Source: CAD feature listing. Evaluate the final solid. Frame: model axes, mm. A direction names the side the tool comes from. Give positions to 0.01 mm unless a question says otherwise; leave off trailing zeros. Order: outer loops, then holes, each group sorted by start corner. A loop starts at its lowest first (then second) coordinate and runs counter-clockwise, first axis right, second up. Notation, with made-up numbers: M 22.25,57 L 40.25,57 A16 cw 40.25,82 Z; hole C 39.25,62.25 d11. An arc over 180 degrees is marked long. Answer as a JSON object with one key per item and string values. Group by question number.
1. Section query C-C (x = 19). Output: boundary loops of the cut face in (y, z).
2. Pin query (flat end, axial travel): P1, Ø5, axis at x = -5.5, y = 4.5, coming from the +Z side. Return the tip coordinate at first contact, or that it passes through.
3. Section query A-A (z = 85.5). Output: boundary loops of the cut face in (x, y).
4. Material intervals for L1, parallel to Y at x = 6, z = 121.5; L2, parallel to X at y = -14.5, z = 15; L3, parallel to Y at x = -23, z = 114, sorted ascending. Write a range as [from, to].
5. Pull-direction query (Y, two-part tool) for faces 3 (the flat face through (0, 29.4, 65)), 4 (the cylindrical face through (-24.607, 29.916, 63.907)), 5 (the conical face through (23.6, 28.814, 128.708)), 6 (the flat face through (-25.75, 0, 64)); classes: +Y half, -Y half, draft (parallel to the pull), parting line (faces both ways), or undercut.
6. Section query B-B (y = -24). Output: boundary loops of the cut face in (x, z).
7. Set-up query: faces 1 (the flat face through (0, 0, 2.6)), 2 (the conical face through (-24.18, 29.47, 0.38)). Return all of +Z, -Z, +X, -X, +Y, -Y with unobstructed straight access to the full face (end or side cutting, diameter ignored); none if empty.
from build123d import *

# Parameters (mm, degrees)
WALLS_DEPTH            = 129
FLOOR_2_DEPTH          = 2.6
BOTTOM_CHAMFERS_SIZE   = 1
TOP_CHAMFERS_SIZE      = 0.4
INSIDE_BOTTOM_FILLET_R = 1


with BuildPart() as part:
    # Sketch1 → Walls (new body)
    with BuildSketch(Plane.XY):
        with BuildLine():
            Line((-25.75, 27.2), (-25.75, -27.2))
            ThreePointArc((-25.75, -27.2), (-24.637005769, -29.887005769), (-21.95, -31))
            Line((-21.95, -31), (21.95, -31))
            ThreePointArc((21.95, -31), (24.637005769, -29.887005769), (25.75, -27.2))
            Line((25.75, -27.2), (25.75, 27.2))
            ThreePointArc((25.75, 27.2), (24.637005769, 29.887005769), (21.95, 31))
            Line((21.95, 31), (-21.95, 31))
            ThreePointArc((-21.95, 31), (-24.637005769, 29.887005769), (-25.75, 27.2))
        make_face()
        with BuildLine():
            Line((-24.15, 27.2), (-24.15, -27.2))
            ThreePointArc((-24.15, -27.2), (-23.505634919, -28.755634919), (-21.95, -29.4))
            Line((-21.95, -29.4), (21.95, -29.4))
            ThreePointArc((21.95, -29.4), (23.505634919, -28.755634919), (24.15, -27.2))
            Line((24.15, -27.2), (24.15, 27.2))
            ThreePointArc((24.15, 27.2), (23.505634919, 28.755634919), (21.95, 29.4))
            Line((21.95, 29.4), (-21.95, 29.4))
            ThreePointArc((-21.95, 29.4), (-23.505634919, 28.755634919), (-24.15, 27.2))
        make_face(mode=Mode.SUBTRACT)
    extrude(amount=WALLS_DEPTH)

    # Sketch2 → Floor 2 (add)
    with BuildSketch(Plane(origin=(0, 0, 0), x_dir=(-1, 0, 0), z_dir=(0, 0, -1))):
        with BuildLine():
            Line((-25.75, 27.2), (-25.75, -27.2))
            ThreePointArc((-25.75, -27.2), (-24.637005769, -29.887005769), (-21.95, -31))
            Line((-21.95, -31), (21.95, -31))
            ThreePointArc((21.95, -31), (24.637005769, -29.887005769), (25.75, -27.2))
            Line((25.75, -27.2), (25.75, 27.2))
            ThreePointArc((25.75, 27.2), (24.637005769, 29.887005769), (21.95, 31))
            Line((21.95, 31), (-21.95, 31))
            ThreePointArc((-21.95, 31), (-24.637005769, 29.887005769), (-25.75, 27.2))
        make_face()
    extrude(amount=-FLOOR_2_DEPTH)

    # Bottom Chamfers
    bottom_chamfers_edges = [part.edges().sort_by_distance(p)[0] for p in [
        (25.75, 0, 0),
        (24.637005769, -29.887005769, 0),
        (0, -31, 0),
        (-24.637005769, -29.887005769, 0),
        (-25.75, 0, 0),
        (-24.637005769, 29.887005769, 0),
        (0, 31, 0),
        (24.637005769, 29.887005769, 0),
    ]]
    chamfer(bottom_chamfers_edges, length=BOTTOM_CHAMFERS_SIZE)

    # Top Chamfers
    top_chamfers_edges = [part.edges().sort_by_distance(p)[0] for p in [
        (-24.637005769, 29.887005769, 129),
        (-25.75, 0, 129),
        (-24.637005769, -29.887005769, 129),
        (0, -31, 129),
        (23.505634919, 28.755634919, 129),
        (0, 29.4, 129),
        (-23.505634919, 28.755634919, 129),
        (-24.15, 0, 129),
        (-23.505634919, -28.755634919, 129),
        (24.637005769, -29.887005769, 129),
        (0, -29.4, 129),
        (23.505634919, -28.755634919, 129),
        (24.15, 0, 129),
        (25.75, 0, 129),
        (24.637005769, 29.887005769, 129),
        (0, 31, 129),
    ]]
    chamfer(top_chamfers_edges, length=TOP_CHAMFERS_SIZE)

    # Inside Bottom Fillet
    inside_bottom_fillet_edges = [part.edges().sort_by_distance(p)[0] for p in [
        (24.15, 0, 2.6),
        (0, 29.4, 2.6),
        (23.505634919, 28.755634919, 2.6),
        (23.505634919, -28.755634919, 2.6),
        (0, -29.4, 2.6),
        (-23.505634919, -28.755634919, 2.6),
        (-24.15, 0, 2.6),
        (-23.505634919, 28.755634919, 2.6),
    ]]
    fillet(inside_bottom_fillet_edges, radius=INSIDE_BOTTOM_FILLET_R)


solid = part.part
Answer sheet:
{
 "1": {"outline": "M -31,1 L -30,0 L 30,0 L 31,1 L 31,128.6 L 30.6,129 L 29.8,129 L 29.4,128.6 L 29.4,3.6 A1 cw 28.4,2.6 L -28.4,2.6 A1 cw -29.4,3.6 L -29.4,128.6 L -29.8,129 L -30.6,129 L -31,128.6 Z"},
 "2": {"P1": "z = 2.6"},
 "3": {"outline": "M -25.75,-27.2 A3.8 ccw -21.95,-31 L 21.95,-31 A3.8 ccw 25.75,-27.2 L 25.75,27.2 A3.8 ccw 21.95,31 L -21.95,31 A3.8 ccw -25.75,27.2 Z; hole M -24.15,-27.2 A2.2 ccw -21.95,-29.4 L 21.95,-29.4 A2.2 ccw 24.15,-27.2 L 24.15,27.2 A2.2 ccw 21.95,29.4 L -21.95,29.4 A2.2 ccw -24.15,27.2 Z"},
 "4": {"L1": "[-31, -29.4], [29.4, 31]", "L2": "[-25.75, -24.15], [24.15, 25.75]", "L3": "[-30.85, -29.13], [29.13, 30.85]"},
 "5": {"face 3": "undercut", "face 4": "+Y half", "face 5": "undercut", "face 6": "draft"},
 "6": {"outline": "M -25.75,1 L -24.75,0 L 24.75,0 L 25.75,1 L 25.75,128.6 L 25.35,129 L 24.55,129 L 24.15,128.6 L 24.15,3.6 A1 cw 23.15,2.6 L -23.15,2.6 A1 cw -24.15,3.6 L -24.15,128.6 L -24.55,129 L -25.35,129 L -25.75,128.6 Z"},
 "7": {"face 1": "+Z", "face 2": "-Z, -X, +Y"}
}
